```python
from build123d import *

# Parameters (mm, degrees)
SKETCH1_W           = 104
SKETCH1_H           = 62
BOSS_EXTRUDE1_DEPTH = 4
CUT_EXTRUDE1_DEPTH  = 10
SKETCH4_R           = 1.75
CUT_EXTRUDE3_DEPTH  = 10


with BuildPart() as part:
    # Sketch1 → Boss-Extrude1 (new body)
    with BuildSketch(Plane.XY):
        Rectangle(SKETCH1_W, SKETCH1_H)
    extrude(amount=BOSS_EXTRUDE1_DEPTH)

    # Sketch2 → Cut-Extrude1 (cut)
    with BuildSketch(Plane(origin=(0, 0, 0), x_dir=(-1, 0, 0), z_dir=(0, 0, -1))):
        Polygon((-37.6, -28), (-37.6, -31), (-42, -31), (-42, -28), (-43.5, -28), (-43.5, -24.8), (-42, -24.8), (-42, -17.8), (-37.6, -17.8), (-37.6, -24.8), (-36.1, -24.8), (-36.1, -28), align=None)
        Polygon((42, -31), (42, -28), (43.5, -28), (43.5, -24.8), (42, -24.8), (42, -17.8), (37.6, -17.8), (37.6, -24.8), (36.1, -24.8), (36.1, -28), (37.6, -28), (37.6, -31), align=None)
        Polygon((-42, 31), (-42, 28), (-43.5, 28), (-43.5, 24.8), (-42, 24.8), (-42, 17.8), (-37.6, 17.8), (-37.6, 24.8), (-36.1, 24.8), (-36.1, 28), (-37.6, 28), (-37.6, 31), align=None)
        Polygon((14.4, 24.8), (14.4, 17.8), (10, 17.8), (10, 24.8), (8.5, 24.8), (8.5, 28), (10, 28), (10, 31), (14.4, 31), (14.4, 28), (15.9, 28), (15.9, 24.8), align=None)
    extrude(amount=-CUT_EXTRUDE1_DEPTH, mode=Mode.SUBTRACT)

    # Sketch4 → Cut-Extrude3 (cut)
    with BuildSketch(Plane(origin=(0, 0, 0), x_dir=(-1, 0, 0), z_dir=(0, 0, -1))):
        with Locations((-26.75, 18.25)):
            Circle(SKETCH4_R)
        with Locations((-26.75, -18.25)):
            Circle(SKETCH4_R)
        with Locations((26.75, 18.25)):
            Circle(SKETCH4_R)
        with Locations((26.75, -19.415816569)):
            Circle(SKETCH4_R)
    extrude(amount=-CUT_EXTRUDE3_DEPTH, mode=Mode.SUBTRACT)


solid = part.part
```
The model under review builds one solid part; all positions refer to its coordinate system, in mm. A direction names the side the tool comes from. Coordinates: 2 decimals unless noted, no trailing zeros. Write each loop counter-clockwise with the first axis right and the second up, starting at its lowest first coordinate (ties: lowest second). Pieces come first, ordered by that corner, then holes. Notation, with made-up numbers: (63, 88.25) -> (67, 88.25) arc R22 ccw to (67, 111.25) -> close; hole circle Ø6 at (-0.75, -2). An arc over 180 degrees is marked (long way). One line per item, written item: value. Start each with the question number.
Q1. For faces 5 (the face through (37.6, -29, 2)), 6 (the face through (-52, 0, 2)), 7 (the face through (-1, 0, 4)), 8 (the face through (42, 21, 2)), 9 (the face through (36.1, 26, 2)), list the 3-axis set-ups (+Z, -Z, +X, -X, +Y, -Y) from which the entire face can be reached by the end or side of a thin tool; tool diameter is ignored.
Q2. Add section B-B, the plane z = 1.5. Count the separate pieces of the cut face and the enclosed holes in it, then the cut area to 3 significant figures.
Q3. Clearance check with a flat-ended pin moving along its axis: P1, Ø2, axis at x = 39.5, z = 2.5, coming from the -Y side. State where the tip first meets the part, or that it passes through.
Q4. Add section A-A, the plane x = 26.75. Give the boundary of the cut face in (y, z).
Q5. The part is to be moulded in two halves that separate along Y. For faces 1 (the face through (28.04, -17.07, 1.97)), 2 (the face through (47, 31, 2)), 3 (the face through (52, 0, 2)), 4 (the face through (-8.5, 26, 2)), say which applies: +Y half, -Y half, draft (parallel to the pull), parting line (faces both ways), or undercut.
Q6. To check wall thickness, follow probe 1 along Y at (x, z) = (26.75, 2.4); probe 2 along Y at (x, z) = (-26.75, 1.6); probe 3 along Y at (x, z) = (-42.5, 1.7). State the ranges of each line that lie inside material, in increasing order.
Response:
1. face 5: +Z, -Z, -Y
1. face 6: +Z, -Z, -X, +Y, -Y
1. face 7: +Z, +X, -X, +Y, -Y
1. face 8: +Z, -Z, +Y
1. face 9: +Z, -Z
2. separate pieces: 1
2. enclosed holes: 4
2. area: 6,140 mm²
3. P1: y = -17.8
4. outline: (-31, 0) -> (-20, 0) -> (-20, 4) -> (-31, 4) -> close; (-16.5, 0) -> (16.5, 0) -> (16.5, 4) -> (-16.5, 4) -> close; (20, 0) -> (31, 0) -> (31, 4) -> (20, 4) -> close
5. face 1: undercut
5. face 2: +Y half
5. face 3: draft
5. face 4: undercut
6. probe 1: -31 to -20, -16.5 to 16.5, 20 to 31
6. probe 2: -31 to -21.17, -17.67 to 16.5, 20 to 31
6. probe 3: -31 to -28, -24.8 to 31
